Autodesk Inventor part; units mm, degrees
ref_plane "YZ Plane" through (0, 0, 0) normal (1, 0, 0) x (0, 1, 0)
ref_plane "XZ Plane" through (0, 0, 0) normal (0, 1, 0) x (-1, 0, 0)
ref_plane "XY Plane" through (0, 0, 0) normal (0, 0, 1) x (1, 0, 0)
sketch "Sketch1" plane through (0, 0, 0) normal (0, 0, 1) x (1, 0, 0)
  line L0 (45, -50) -> (-45, -50)
  line L1 (-45, -50) -> (-45, 50)
  line L2 (-45, 50) -> (45, 50)
  line L3 (45, 50) -> (45, -50)
  line L4 (45, -50) -> (-45, 50) construction
  line L5 (-45, -50) -> (45, 50) construction
  line L6 (53, 58) -> (-53, 58)
  line L7 (-53, 58) -> (-53, 54.5)
  line L8 (-53, -58) -> (53, -58)
  line L9 (53, -58) -> (53, -54.5)
  line L10 (-20, 50) -> (20, 50)
  line L11 (-20, -50) -> (20, -50)
  line L12 (-45, -20) -> (-45, 20)
  line L13 (45, -20) -> (45, 20)
  line L14 (-53, 6.5) -> (-77, 6.5)
  line L15 (-53, -6.5) -> (-53, 6.5) construction
  line L16 (-53, 0) -> (53, 0)
  line L17 (0, 50) -> (0, -50)
  line L18 (-53, 6.5) -> (-53, -6.5) construction
  line L19 (-53, -6.5) -> (-53, -44.5)
  line L20 (53, 6.5) -> (53, 44.5)
  line L21 (53, -6.5) -> (53, 6.5) construction
  line L22 (-92, -6.5) -> (-77, -6.5) construction
  line L23 (-77, -6.5) -> (-77, -44.5)
  line L24 (-77, -58) -> (-92, -58) construction
  line L25 (-92, -58) -> (-92, -54.5) construction
  line L26 (-92, -58) -> (-77, -58) construction
  line L27 (-77, -58) -> (-77, -58.5) construction
  line L28 (-77, -58.5) -> (-81.5, -58.5) construction
  line L29 (-92, -58.5) -> (-92, -58) construction
  line L30 (-92, -54.5) -> (-87.5, -54.5)
  line L31 (-87.5, -54.5) -> (-87.5, -58.5)
  line L32 (-81.5, -58.5) -> (-81.5, -54.5)
  line L33 (-81.5, -54.5) -> (-77, -54.5)
  line L34 (-77, 6.5) -> (-77, 44.5)
  line L35 (-77, 58) -> (-92, 58) construction
  line L36 (-92, 58) -> (-92, 54.5) construction
  line L37 (-92, 58) -> (-77, 58) construction
  line L38 (-77, 58) -> (-77, 58.5) construction
  line L39 (-77, 58.5) -> (-81.5, 58.5) construction
  line L40 (-92, 58.5) -> (-92, 58) construction
  line L41 (-92, 54.5) -> (-87.5, 54.5)
  line L42 (-87.5, 54.5) -> (-87.5, 58.5)
  line L43 (-81.5, 58.5) -> (-81.5, 54.5)
  line L44 (-81.5, 54.5) -> (-77, 54.5)
  line L45 (-77, 6.5) -> (-92, 6.5) construction
  line L46 (-92, -6.5) -> (-77, -6.5) construction
  line L47 (-77, -6.5) -> (-53, -6.5)
  line L48 (-77, 54.5) -> (-77, 58) construction
  line L49 (-92, 54.5) -> (-92, 6.5)
  line L50 (-87.5, 58.5) -> (-92, 58.5) construction
  line L51 (-81.5, 58.5) -> (-87.5, 58.5)
  line L52 (-92, -54.5) -> (-92, -6.5)
  line L53 (-87.5, -58.5) -> (-92, -58.5) construction
  line L54 (-81.5, -58.5) -> (-87.5, -58.5)
  line L55 (-77, -54.5) -> (-77, -58) construction
  line L56 (-77, 54.5) -> (-71.5, 54.5)
  line L57 (-53, 54.5) -> (-53, 44.5) construction
  line L58 (-53, 44.5) -> (-77, 44.5)
  line L59 (-77, 44.5) -> (-77, 54.5) construction
  line L60 (-77, -54.5) -> (-71.5, -54.5)
  line L61 (-53, -54.5) -> (-53, -54)
  line L62 (-53, -44.5) -> (-77, -44.5)
  line L63 (-77, -44.5) -> (-77, -54.5) construction
  line L64 (-71.5, 54.5) -> (-65.5, 54.5) construction
  line L65 (-65.5, 54.5) -> (-65.5, 58.5)
  line L66 (-65.5, 58.5) -> (-71.5, 58.5)
  line L67 (-71.5, 58.5) -> (-71.5, 54.5)
  line L68 (-71.5, -54.5) -> (-65.5, -54.5) construction
  line L69 (-65.5, -54.5) -> (-65.5, -58.5)
  line L70 (-65.5, -58.5) -> (-71.5, -58.5)
  line L71 (-71.5, -58.5) -> (-71.5, -54.5)
  line L72 (-71.5, 54.5) -> (-65.5, 54.5) construction
  line L73 (-65.5, 54.5) -> (-53, 54.5)
  line L74 (-77, 44.5) -> (-77, 54.5) construction
  line L75 (-53, 44.5) -> (-53, 6.5)
  line L76 (-53, 54.5) -> (-53, 44.5) construction
  line L77 (-77, -44.5) -> (-77, -54.5) construction
  line L78 (-53, -44.5) -> (-53, -54.5) construction
  line L79 (-53, -54) -> (-53, -44.5) construction
  line L80 (-65.5, -54.5) -> (-53, -54.5)
  line L81 (-71.5, -54.5) -> (-65.5, -54.5) construction
  line L82 (-53, -54.5) -> (-53, -58)
  line L83 (53, 6.5) -> (77, 6.5)
  line L84 (92, -6.5) -> (77, -6.5) construction
  line L85 (77, -6.5) -> (77, -44.5)
  line L86 (77, -58) -> (92, -58) construction
  line L87 (92, -58) -> (92, -54.5) construction
  line L88 (92, -58) -> (77, -58) construction
  line L89 (77, -58) -> (77, -58.5) construction
  line L90 (77, -58.5) -> (81.5, -58.5) construction
  line L91 (92, -58.5) -> (92, -58) construction
  line L92 (92, -54.5) -> (87.5, -54.5)
  line L93 (87.5, -54.5) -> (87.5, -58.5)
  line L94 (81.5, -58.5) -> (81.5, -54.5)
  line L95 (81.5, -54.5) -> (77, -54.5)
  line L96 (92, 54.5) -> (87.5, 54.5)
  line L97 (92, 58) -> (92, 54.5) construction
  line L98 (77, 6.5) -> (77, 44.5)
  line L99 (81.5, 54.5) -> (77, 54.5)
  line L100 (77, 58) -> (92, 58) construction
  line L101 (92, 58) -> (77, 58) construction
  line L102 (77, 58) -> (77, 58.5) construction
  line L103 (77, 58.5) -> (81.5, 58.5) construction
  line L104 (81.5, 58.5) -> (81.5, 54.5)
  line L105 (92, 58.5) -> (92, 58) construction
  line L106 (87.5, 54.5) -> (87.5, 58.5)
  line L107 (77, 6.5) -> (92, 6.5) construction
  line L108 (92, -6.5) -> (77, -6.5) construction
  line L109 (77, -6.5) -> (53, -6.5)
  line L110 (77, 54.5) -> (77, 58) construction
  line L111 (92, 54.5) -> (92, 6.5)
  line L112 (87.5, 58.5) -> (92, 58.5) construction
  line L113 (81.5, 58.5) -> (87.5, 58.5)
  line L114 (92, -54.5) -> (92, -6.5)
  line L115 (87.5, -58.5) -> (92, -58.5) construction
  line L116 (81.5, -58.5) -> (87.5, -58.5)
  line L117 (77, -54.5) -> (77, -58) construction
  line L118 (77, 54.5) -> (71.5, 54.5)
  line L119 (53, 44.5) -> (77, 44.5)
  line L120 (77, 44.5) -> (77, 54.5) construction
  line L121 (77, -54.5) -> (71.5, -54.5)
  line L122 (53, -44.5) -> (77, -44.5)
  line L123 (77, -44.5) -> (77, -54.5) construction
  line L124 (71.5, 54.5) -> (65.5, 54.5) construction
  line L125 (65.5, 54.5) -> (65.5, 58.5)
  line L126 (65.5, 58.5) -> (71.5, 58.5)
  line L127 (71.5, 58.5) -> (71.5, 54.5)
  line L128 (71.5, -54.5) -> (65.5, -54.5) construction
  line L129 (65.5, -54.5) -> (65.5, -58.5)
  line L130 (65.5, -58.5) -> (71.5, -58.5)
  line L131 (71.5, -58.5) -> (71.5, -54.5)
  line L132 (71.5, 54.5) -> (65.5, 54.5) construction
  line L133 (65.5, 54.5) -> (53, 54.5)
  line L134 (77, 44.5) -> (77, 54.5) construction
  line L135 (77, -44.5) -> (77, -54.5) construction
  line L136 (65.5, -54.5) -> (53, -54.5)
  line L137 (71.5, -54.5) -> (65.5, -54.5) construction
  line L138 (53, 44.5) -> (53, 54.5) construction
  line L139 (53, 54.5) -> (53, 58)
  line L140 (53, -44.5) -> (53, -6.5)
  line L141 (53, -54.5) -> (53, -44.5) construction
  line L142 (-92, 6.5) -> (-92, -6.5)
  line L143 (92, 6.5) -> (92, -6.5)
  point P0 (0, 0)
  point P1 (0, 54)
  point P2 (0, 0)
  point P3 (-49, 0)
  point P4 (0, 0)
  point P5 (-53, 0)
  point P6 (0, 0)
  point P7 (0, 0)
  point P8 (-84.5, -58)
  point P9 (-84.5, 58)
  point P10 (-65, 44.5)
  point P11 (-81.5, 56.5)
  point P12 (-71.5, 56.5)
  point P13 (84.5, -58)
  point P14 (84.5, 58)
  point P15 (65, 44.5)
  point P16 (81.5, 56.5)
  point P17 (71.5, 56.5)
  dimension "d0" = 100
  dimension "d1" = 90
  dimension "d2" = 8
  dimension "d16" = 15
  dimension "d17" = 0.5
  dimension "d18" = 6
  dimension "d19" = 4.5
  dimension "d20" = 4.5
  dimension "d21" = 4
  dimension "d24" = 10
  dimension "d25" = 10
  dimension "d27" = 10
  dimension "d28" = 6
  dimension "d29" = 8
  dimension "d30" = 8
  dimension "d31" = 4.5
  dimension "d32" = 24
extrude "Extrusion1" add sketch "Sketch1" along normal blind 4
properties part number "DoorFrameFront_V2" material "Wood (Oak)"
Here's how the part is built. I have some questions about the finished solid (model axes, mm). A direction names the side the tool comes from. Round coordinates to 2 decimals unless told otherwise and drop trailing zeros. Write each loop counter-clockwise with the first axis right and the second up, starting at its lowest first coordinate (ties: lowest second). Pieces come first, ordered by that corner, then holes.
Q1. Will these pins go through, and if not, where does the flat tip stop? P1, Ø1.2, axis at y = 56.5, z = 2, coming from the +X side; P2, Ø1.5, axis at x = 21.5, z = 3, coming from the +Y side; P3, Ø1, axis at x = 59.5, z = 1, coming from the +Y side.
Q2. If we section it at C-C on y = -1: Write out the boundary of the cut face in (x, z).
Q3. Which directions (+Z, -Z, +X, -X, +Y, -Y) give clear straight access to the entire face, cutting with the end or side of a thin tool? Please do faces 1 (the flat face through (-71.5, -57, 2)), 2 (the flat face through (90, 54.5, 2)), 3 (the flat face through (65, -6.5, 2)), 4 (the flat face through (65.5, 56, 2)), 5 (the flat face through (-92, 1, 2)).
Q4. If we section it at B-B on x = -56.5: Write out the boundary of the cut face in (y, z).
Q5. If we section it at D-D on x = 31.5: Write out the boundary of the cut face in (y, z).
Q6. If we mould it in two halves opening along X, with no side actions, what happens to faces 6 (the flat face through (-65.5, -56, 2)), 7 (the flat face through (-90, 54.5, 2)), 8 (the flat face through (87.5, 56, 2))? For each: +X half, -X half, draft (parallel to the pull), parting line (faces both ways), or undercut.
Q7. If we section it at A-A on y = 20: Write out the boundary of the cut face in (x, z).
Q8. Please list where these lines run through material, in increasing order: probe 1 along X at (y, z) = (11.5, 1.95); probe 2 along Y at (x, z) = (-16, 2.4); probe 3 along X at (y, z) = (6, 0.8).
Answer below:
1. P1: stops at x = 87.5
1. P2: stops at y = 58
1. P3: stops at y = 54.5
2. outline: (-92, 0) - (-45, 0) - (-45, 4) - (-92, 4) - close; (45, 0) - (92, 0) - (92, 4) - (45, 4) - close
3. face 1: +Z, -Z, -Y
3. face 2: +Z, -Z, +X, +Y
3. face 3: +Z, -Z
3. face 4: +Z, -Z, +Y
3. face 5: +Z, -Z, -X, +Y, -Y
4. outline: (-54.5, 0) - (-44.5, 0) - (-44.5, 4) - (-54.5, 4) - close; (-6.5, 0) - (6.5, 0) - (6.5, 4) - (-6.5, 4) - close; (44.5, 0) - (54.5, 0) - (54.5, 4) - (44.5, 4) - close
5. outline: (-58, 0) - (-50, 0) - (-50, 4) - (-58, 4) - close; (50, 0) - (58, 0) - (58, 4) - (50, 4) - close
6. face 6: undercut
6. face 7: draft
6. face 8: +X half
7. outline: (-92, 0) - (-77, 0) - (-77, 4) - (-92, 4) - close; (-53, 0) - (-45, 0) - (-45, 4) - (-53, 4) - close; (45, 0) - (53, 0) - (53, 4) - (45, 4) - close; (77, 0) - (92, 0) - (92, 4) - (77, 4) - close
8. probe 1: x = -92 to -77, -53 to -45, 45 to 53, 77 to 92
8. probe 2: y = -58 to -50, 50 to 58
8. probe 3: x = -92 to -45, 45 to 92
